Geometry: final body of the model. Coordinates: model frame, mm. Face numbers are marked on the shaded views. Coordinates: 2 decimals unless noted, no trailing zeros. Loops run counter-clockwise (first coordinate to the right, second up) from the corner with the lowest first, then second, coordinate; pieces in that order, holes last. Notation, with made-up numbers: (-5.75, -33) -> (5.25, -33) arc R22 ccw to (5.25, -6) -> close; hole circle Ø7 at (35.25, 81.25). An arc over 180 degrees is marked (long way). One line per item, written item: value. Start each with the question number.
Autodesk Inventor part; units mm, degrees
ref_plane "YZ Plane" through (0, 0, 0) normal (1, 0, 0) x (0, 1, 0)
ref_plane "XZ Plane" through (0, 0, 0) normal (0, 1, 0) x (-1, 0, 0)
ref_plane "XY Plane" through (0, 0, 0) normal (0, 0, 1) x (1, 0, 0)
sketch "スケッチ1" plane through (0, 0, 0) normal (0, 0, 1) x (1, 0, 0)
  circle A0 centre (0, 0) radius 20.5
  circle A1 centre (0, 0) radius 10 construction
  circle A2 centre (0, 0) radius 7 construction
  circle A3 centre (0, -7) radius 1.1
  circle A4 centre (4.9497, -4.9497) radius 1.1
  circle A5 centre (7, 0) radius 1.1
  circle A6 centre (4.9497, 4.9497) radius 1.1
  circle A7 centre (0, 7) radius 1.1
  circle A8 centre (-4.9497, 4.9497) radius 1.1
  circle A9 centre (-7, 0) radius 1.1
  circle A10 centre (-4.9497, -4.9497) radius 1.1
  circle A11 centre (0, 0) radius 15.5 construction
  circle A12 centre (0, 0) radius 12 construction
  line L0 (0, -12) -> (0, -15.5) construction
  circle A13 centre (0, -13.75) radius 1.25
  circle A14 centre (43.1211, 8.0958) radius 5
  circle A15 centre (46.9662, 2.2465) radius 0.8
  circle A16 centre (49.9761, 6.6786) radius 0.8
  circle A17 centre (48.9705, 11.9409) radius 0.8
  circle A18 centre (44.5383, 14.9509) radius 0.8
  circle A19 centre (39.276, 13.9452) radius 0.8
  circle A20 centre (36.2661, 9.513) radius 0.8
  circle A21 centre (37.2717, 4.2507) radius 0.8
  circle A22 centre (41.7039, 1.2408) radius 0.8
  circle A23 centre (43.1211, 8.0958) radius 10
  circle A24 centre (0, 0) radius 5.1
  circle A25 centre (0, 0) radius 13.75 construction
  circle A26 centre (9.7227, -9.7227) radius 1.25
  circle A27 centre (13.75, 0) radius 1.25
  circle A28 centre (9.7227, 9.7227) radius 1.25
  circle A29 centre (0, 13.75) radius 1.25
  circle A30 centre (-9.7227, 9.7227) radius 1.25
  circle A31 centre (-13.75, 0) radius 1.25
  circle A32 centre (-9.7227, -9.7227) radius 1.25
  dimension "d2" = 14
  dimension "d6" = 360
  dimension "d0" = 41
  dimension "d1" = 20
  dimension "d3" = 2.2
  dimension "d8" = 5
  dimension "d10" = 2.5
  dimension "d15" = 10.2
  dimension "d18" = 27.5
  dimension "d19" = 13.75
  dimension "d22" = 360
extrude "押し出し2" add sketch "スケッチ1" along normal blind 3 contours A0
properties part number "出力部品A_ダブルスラスト用(t2_アルミ)" material "アルミニウム 6061"
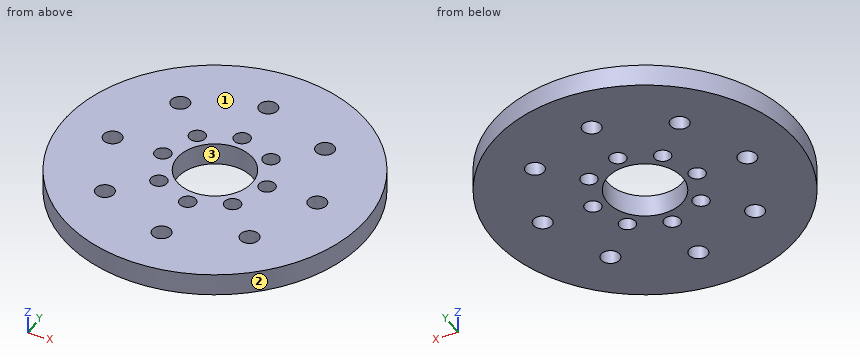
1. Section A-A on y = 0. Return the cut outline in (x, z).
2. Section C-C on z = 1.5. Count the separate pieces of the cut face and the enclosed holes in it, plus the area to 3 significant figures.
3. Pin query (flat end, axial travel): pin 1 Ø2 at (x, y) = (-7, 0) entering from +Z; pin 2 Ø1 at (x, z) = (-4.5, 2) entering from -Y. Return the tip coordinate at first contact, or that it passes through.
4. Draft query along X for the marked faces 1, 2 and 3. Return one class per face: released by +X, released by -X, zero draft, split by the parting line, or undercut.
5. Line query: L1, parallel to X at y = 4.5, z = 0.2; L2, parallel to Y at x = 4, z = 1.3; L3, parallel to X at y = -1, z = 1.95. Output: solid intervals per line, ascending. Write a range as [from, to].
6. Section D-D on x = -7. Return the cut outline in (y, z).
Checks:
1. outline: (-20.5, 0) -> (-15, 0) -> (-15, 3) -> (-20.5, 3) -> close; (-12.5, 0) -> (-8.1, 0) -> (-8.1, 3) -> (-12.5, 3) -> close; (-5.9, 0) -> (-5.1, 0) -> (-5.1, 3) -> (-5.9, 3) -> close; (5.1, 0) -> (5.9, 0) -> (5.9, 3) -> (5.1, 3) -> close; (8.1, 0) -> (12.5, 0) -> (12.5, 3) -> (8.1, 3) -> close; (15, 0) -> (20.5, 0) -> (20.5, 3) -> (15, 3) -> close
2. separate pieces: 1
2. enclosed holes: 17
2. area: 1,170 mm²
3. pin 1: through
3. pin 2: y = -20.11
4. face 1: zero draft
4. face 2: split by the parting line
4. face 3: undercut
5. L1: [-20, -5.95], [-3.95, -2.4], [2.4, 3.95], [5.95, 20]
5. L2: [-20.11, -5.5], [-4.39, -3.16], [3.16, 4.39], [5.5, 20.11]
5. L3: [-20.48, -14.5], [-13, -7.46], [-6.54, -5], [5, 6.54], [7.46, 13], [14.5, 20.48]
6. outline: (-19.27, 0) -> (-1.1, 0) -> (-1.1, 3) -> (-19.27, 3) -> close; (1.1, 0) -> (19.27, 0) -> (19.27, 3) -> (1.1, 3) -> close
